from build123d import *

# Parameters (mm, degrees)
F0_W     = 80
F0_H     = 107
F0_R     = 2.5
F0_W_2   = 34.5
F0_H_2   = 76.5
F0_R_2   = 4.25
F1_DEPTH = 15
F2_W     = 80
F2_H     = 107
F3_DEPTH = 2
F4_R     = 5


with BuildPart() as f1:
    # F0 (on Top) → F1 (new body)
    with BuildSketch(Plane.XY):
        with Locations((40, 53.5)):
            Rectangle(F0_W, F0_H)
        with Locations((5, 5)):
            Circle(F0_R, mode=Mode.SUBTRACT)
        with Locations((5, 13)):
            Circle(F0_R, mode=Mode.SUBTRACT)
        with Locations((13, 5)):
            Circle(F0_R, mode=Mode.SUBTRACT)
        with Locations((13, 13)):
            Circle(F0_R, mode=Mode.SUBTRACT)
        with Locations((5, 21)):
            Circle(F0_R, mode=Mode.SUBTRACT)
        with Locations((13, 21)):
            Circle(F0_R, mode=Mode.SUBTRACT)
        with Locations((21, 5)):
            Circle(F0_R, mode=Mode.SUBTRACT)
        with Locations((29, 5)):
            Circle(F0_R, mode=Mode.SUBTRACT)
        with Locations((21, 13)):
            Circle(F0_R, mode=Mode.SUBTRACT)
        with Locations((29, 13)):
            Circle(F0_R, mode=Mode.SUBTRACT)
        with Locations((37, 5)):
            Circle(F0_R, mode=Mode.SUBTRACT)
        with Locations((37, 13)):
            Circle(F0_R, mode=Mode.SUBTRACT)
        with Locations((21, 21)):
            Circle(F0_R, mode=Mode.SUBTRACT)
        with Locations((29, 21)):
            Circle(F0_R, mode=Mode.SUBTRACT)
        with Locations((37, 21)):
            Circle(F0_R, mode=Mode.SUBTRACT)
        with Locations((5, 29)):
            Circle(F0_R, mode=Mode.SUBTRACT)
        with Locations((5, 37)):
            Circle(F0_R, mode=Mode.SUBTRACT)
        with Locations((13, 29)):
            Circle(F0_R, mode=Mode.SUBTRACT)
        with Locations((13, 37)):
            Circle(F0_R, mode=Mode.SUBTRACT)
        with Locations((5, 45)):
            Circle(F0_R, mode=Mode.SUBTRACT)
        with Locations((5, 53)):
            Circle(F0_R, mode=Mode.SUBTRACT)
        with Locations((13, 45)):
            Circle(F0_R, mode=Mode.SUBTRACT)
        with Locations((13, 53)):
            Circle(F0_R, mode=Mode.SUBTRACT)
        with Locations((21, 29)):
            Circle(F0_R, mode=Mode.SUBTRACT)
        with Locations((29, 29)):
            Circle(F0_R, mode=Mode.SUBTRACT)
        with Locations((21, 37)):
            Circle(F0_R, mode=Mode.SUBTRACT)
        with Locations((29, 37)):
            Circle(F0_R, mode=Mode.SUBTRACT)
        with Locations((37, 29)):
            Circle(F0_R, mode=Mode.SUBTRACT)
        with Locations((37, 37)):
            Circle(F0_R, mode=Mode.SUBTRACT)
        with Locations((21, 45)):
            Circle(F0_R, mode=Mode.SUBTRACT)
        with Locations((29, 45)):
            Circle(F0_R, mode=Mode.SUBTRACT)
        with Locations((21, 53)):
            Circle(F0_R, mode=Mode.SUBTRACT)
        with Locations((29, 53)):
            Circle(F0_R, mode=Mode.SUBTRACT)
        with Locations((37, 45)):
            Circle(F0_R, mode=Mode.SUBTRACT)
        with Locations((37, 53)):
            Circle(F0_R, mode=Mode.SUBTRACT)
        with Locations((59.75, 41)):
            Rectangle(F0_W_2, F0_H_2, mode=Mode.SUBTRACT)
        with Locations((5, 61)):
            Circle(F0_R, mode=Mode.SUBTRACT)
        with Locations((13, 61)):
            Circle(F0_R, mode=Mode.SUBTRACT)
        with Locations((5, 69)):
            Circle(F0_R, mode=Mode.SUBTRACT)
        with Locations((5, 77)):
            Circle(F0_R, mode=Mode.SUBTRACT)
        with Locations((13, 69)):
            Circle(F0_R, mode=Mode.SUBTRACT)
        with Locations((13, 77)):
            Circle(F0_R, mode=Mode.SUBTRACT)
        with Locations((21, 61)):
            Circle(F0_R, mode=Mode.SUBTRACT)
        with Locations((29, 61)):
            Circle(F0_R, mode=Mode.SUBTRACT)
        with Locations((37, 61)):
            Circle(F0_R, mode=Mode.SUBTRACT)
        with Locations((21, 69)):
            Circle(F0_R, mode=Mode.SUBTRACT)
        with Locations((29, 69)):
            Circle(F0_R, mode=Mode.SUBTRACT)
        with Locations((21, 77)):
            Circle(F0_R, mode=Mode.SUBTRACT)
        with Locations((29, 77)):
            Circle(F0_R, mode=Mode.SUBTRACT)
        with Locations((37, 69)):
            Circle(F0_R, mode=Mode.SUBTRACT)
        with Locations((37, 77)):
            Circle(F0_R, mode=Mode.SUBTRACT)
        with Locations((15, 92)):
            Circle(F0_R_2, mode=Mode.SUBTRACT)
        with Locations((40, 92)):
            Circle(F0_R_2, mode=Mode.SUBTRACT)
        with Locations((65, 92)):
            Circle(F0_R_2, mode=Mode.SUBTRACT)
    extrude(amount=F1_DEPTH)

    # F2 (on face) → F3 (join)
    with BuildSketch(Plane(origin=(0, 0, 0), x_dir=(1, 0, 0), z_dir=(0, 0, -1))):
        with Locations((40, -53.5)):
            Rectangle(F2_W, F2_H)
    extrude(amount=-F3_DEPTH)

    # F4
    f4_edges = [f1.edges().sort_by_distance(p)[0] for p in [
        (0, 107, 7.5),
        (0, 0, 7.5),
        (80, 0, 7.5),
        (80, 107, 7.5),
    ]]
    fillet(f4_edges, radius=F4_R)


solid = f1.part
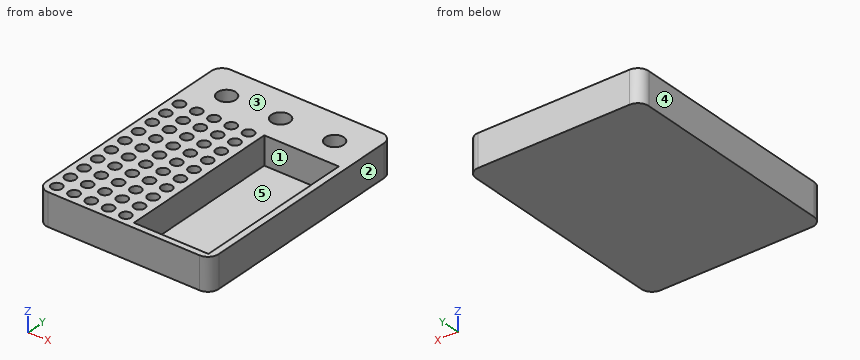
The listing builds one solid part. Answer for the finished solid, in the listing's coordinates (mm). Face numbers are marked on the shaded views. A direction names the side the tool comes from. Give positions to 0.01 mm unless a question says otherwise; leave off trailing zeros. Order: outer loops, then holes, each group sorted by start corner. A loop starts at its lowest first (then second) coordinate and runs counter-clockwise, first axis right, second up. Notation, with made-up numbers: (81, 84.5) - (109, 84.5) arc R10 cw to (109, 93.5) - close; hole circle Ø10 at (89.5, 43). An arc over 180 degrees is marked (long way). Use one line per item in the form item = value.
1) For the marked faces 1 and 2, determine the directions among +Z, -Z, +X, -X, +Y, -Y from which every point of the face is accessible in a straight line to the end or side of a thin tool.
Verdict:
face_1 = +Z
face_2 = +Z, -Z, +X, +Y, -Y
2) The mould has two halves that part along X. Classify the marked faces 3, 4 and 5: released by +X, released by -X, zero draft, split by the parting line, or undercut.
Verdict:
face_3 = zero draft
face_4 = released by -X
face_5 = undercut
3) Each of these flat-tipped pins is pushed along its axis until it touches: pin 1 (5 mm diameter, centred on x = 30.5, y = 25, fed in from -Z); pin 2 (1.5 mm diameter, centred on x = 5, y = 20.5, fed in from +Z). Where does it stop, or does it pass through?
Verdict:
pin_1 = 0
pin_2 = 2
4) Find section B-B on x = 65. Determine the outline of the cut face in (y, z).
Verdict:
outline = (0, 0) - (107, 0) - (107, 15) - (96.25, 15) - (96.25, 2) - (87.75, 2) - (87.75, 15) - (79.25, 15) - (79.25, 2) - (2.75, 2) - (2.75, 15) - (0, 15) - close
5) Find section C-C on z = 3.75. Give the number of separate pieces and of enclosed holes in the cut face, and give its area (3 significant figures).
Verdict:
separate_pieces = 1
enclosed_holes = 54
area = 4,750 mm^2
6) Find section A-A on y = 37. Determine the outline of the cut face in (x, z), and give its area (4 significant figures).
Verdict:
outline = (0, 0) - (80, 0) - (80, 15) - (77, 15) - (77, 2) - (42.5, 2) - (42.5, 15) - (39.5, 15) - (39.5, 2) - (34.5, 2) - (34.5, 15) - (31.5, 15) - (31.5, 2) - (26.5, 2) - (26.5, 15) - (23.5, 15) - (23.5, 2) - (18.5, 2) - (18.5, 15) - (15.5, 15) - (15.5, 2) - (10.5, 2) - (10.5, 15) - (7.5, 15) - (7.5, 2) - (2.5, 2) - (2.5, 15) - (0, 15) - close
area = 426.5 mm^2
7) Consider probe 1 along Y at (x, z) = (60, 11.5); probe 2 along Y at (x, z) = (65, 7.25); probe 3 along X at (y, z) = (66, 11.25). Determine where each line is inside the solid, lowest interval first. Write a range as [from, to].
Verdict:
probe_1 = [0, 2.75], [79.25, 107]
probe_2 = [0, 2.75], [79.25, 87.75], [96.25, 107]
probe_3 = [0, 42.5], [77, 80]
8) Find section D-D on x = 73. Determine the outline of the cut face in (y, z).
Verdict:
outline = (0, 0) - (107, 0) - (107, 15) - (79.25, 15) - (79.25, 2) - (2.75, 2) - (2.75, 15) - (0, 15) - close
